```python
from build123d import *

# Parameters (mm, degrees)
SKETCH_2_W          = 4.25
SKETCH_2_H          = 5
SKETCH_3_R          = 2.5
EXTRUDE_1_DEPTH     = 6
CUT_EXTRUDE_1_DEPTH = 1


with BuildPart() as part:
    # 草图2 → 旋转1 (revolve)
    with BuildSketch(Plane(origin=(0, 0, 0), x_dir=(-1, 0, 0), z_dir=(0, 0, -1)), mode=Mode.PRIVATE) as revolve_1_sk:
        with Locations((-2.125, -2.5)):
            Rectangle(SKETCH_2_W, SKETCH_2_H)
    revolve(revolve_1_sk.sketch.rotate(Axis((0, -5, 0), (0, 1, 0)), 270), axis=Axis((0, -5, 0), (0, 1, 0)))

    # 草图3 → 凸台-拉伸1 (add)
    with BuildSketch(Plane(origin=(0, 0, 0), x_dir=(-1, 0, 0), z_dir=(0, 1, 0))):
        with Locations(Location((0, 0, 0), (0, 0, 90))):
            Circle(SKETCH_3_R)
    extrude(amount=EXTRUDE_1_DEPTH)

    # 草图4 → 切除-拉伸1 (cut)
    with BuildSketch(Plane.XZ.offset(5)):
        Polygon((-1.154700538, -2), (1.154700538, -2), (2.309401077, 0), (1.154700538, 2), (-1.154700538, 2), (-2.309401077, 0), align=None)
    extrude(amount=-CUT_EXTRUDE_1_DEPTH, mode=Mode.SUBTRACT)


solid = part.part
```
Geometry check sheet. Reference: the model listing, model coordinates, mm. A direction names the side the tool comes from. Coordinates: 2 decimals unless noted, no trailing zeros. Write each loop counter-clockwise with the first axis right and the second up, starting at its lowest first coordinate (ties: lowest second). Pieces come first, ordered by that corner, then holes. Notation, with made-up numbers: M 8.5,78.25 L 18.5,78.25 A17 ccw 18.5,94.25 Z; hole C -8,85.5 d3. An arc over 180 degrees is marked long. One line per item, written item: value. Start each with the question number.
(1) Sectioned sample at A-A, the plane x = 0. Enter the section's corners in (y, z).
(2) Release check for a two-part mould opening along Z. For faces 1 (the face through (1.724, -4.507, -1.014)), 2 (the face through (-2.44, 2.96, -0.54)), 3 (the face through (-1.724, -4.507, 1.014)), 4 (the face through (-2, -5, 1)) record: released by +Z, released by -Z, zero draft, split by the parting line, or undercut.
(3) Depth check by flat-ended pin: pin 1 (1.2 mm diameter, centred on x = -0.5, z = -1, fed in from -Y); pin 2 (1.1 mm diameter, centred on x = 0.5, y = -4.5, fed in from +Z); pin 3 (2 mm diameter, centred on y = -3.5, z = 3, fed in from +X); pin 4 (1 mm diameter, centred on x = -3, y = -2, fed in from -Z). Enter the tip coordinate at first touch or a pass-through.
(4) Sectioned sample at C-C, the plane y = 0.75. Enter the section's corners in (x, z).
(5) Sectioned sample at B-B, the plane z = 1.5. Enter the section's corners in (x, y), and give its area (3 significant figures).
(6) Tool access check on faces 5 (the face through (-2, 0, 2)), 6 (the face through (0, 6, 0)), 7 (the face through (1.74, -4.51, 0.99)). Record the directions out of +Z, -Z, +X, -X, +Y, -Y that give a thin tool (end or side, any length) a straight path to the whole face; none if there is none.
(7) Sectioned sample at D-D, the plane y = -1. Enter the section's corners in (x, z).
(8) Scan lines: line 1 along Y through (x, z) = (-0.25, -1.75); line 2 along Y through (x, z) = (3.5, -1.75); line 3 along X through (y, z) = (2.75, -1.5). Record each from-to range of solid material in increasing order. Write a range as [from, to].
Filled sheet:
1. outline: M -5,-4.25 L 0,-4.25 L 0,-2.5 L 6,-2.5 L 6,2.5 L 0,2.5 L 0,4.25 L -5,4.25 L -5,2 L -4,2 L -4,-2 L -5,-2 Z
2. face 1: undercut
2. face 2: split by the parting line
2. face 3: undercut
2. face 4: zero draft
3. pin 1: y = -4
3. pin 2: z = 4.25
3. pin 3: x = 3.75
3. pin 4: z = -3.44
4. outline: C 0,0 d5
5. outline: M -3.98,-5 L -1.44,-5 L -1.44,-4 L 1.44,-4 L 1.44,-5 L 3.98,-5 L 3.98,0 L 2,0 L 2,6 L -2,6 L -2,0 L -3.98,0 Z
5. area: 60.9 mm²
6. face 5: +Y
6. face 6: +Z, -Z, +X, -X, +Y
6. face 7: -Y
7. outline: C 0,0 d8.5
8. line 1: [-4, 6]
8. line 2: [-5, 0]
8. line 3: [-2, 2]
